Autodesk Inventor part; units mm, degrees
ref_plane "YZ Plane" through (0, 0, 0) normal (1, 0, 0) x (0, 1, 0)
ref_plane "XZ Plane" through (0, 0, 0) normal (0, 1, 0) x (-1, 0, 0)
ref_plane "XY Plane" through (0, 0, 0) normal (0, 0, 1) x (1, 0, 0)
sketch "Sketch1" plane through (0, 0, 0) normal (0, 1, 0) x (-1, 0, 0)
  circle A0 centre (0, 0) radius 2.54
  circle A1 centre (0, 0) radius 5.461
  dimension "d0" = 5.08
  dimension "d1" = 10.922
extrude "Extrusion1" add sketch "Sketch1" along normal blind 14.605 contours A0 | A1
sketch "Sketch2" plane through (0, 0, 0) normal (1, 0, 0) x (0, 1, 0)
  arc A0 (12.065, -2.54) -> (12.065, 2.54) centre (12.065, 0) ccw
  line L0 (0, 5.461) -> (14.605, 5.461)
  line L1 (0, -5.461) -> (14.605, -5.461)
  line L2 (12.065, 2.54) -> (7.1656, 2.54)
  line L3 (12.065, -2.54) -> (7.1656, -2.54)
  line L4 (4.6256, 5.461) -> (4.6256, 5.08)
  line L5 (4.6256, -5.08) -> (4.6256, -5.461)
  arc A1 (4.6256, 5.08) -> (7.1656, 2.54) centre (7.1656, 5.08) ccw
  arc A2 (7.1656, -2.54) -> (4.6256, -5.08) centre (7.1656, -5.08) ccw
  line L6 (14.605, 2.54) -> (14.605, -2.54)
  line L7 (14.605, -5.461) -> (14.605, 5.461)
  point P0 (0, 0)
  point P1 (14.605, 0)
  dimension "d4" = 2.54
  dimension "d5" = 2.54
extrude "Extrusion2" cut sketch "Sketch2" along normal mid plane 14.605
properties part number "Half Universal"
Verification items for the finished model (mm, model axes). A direction names the side the tool comes from. Round coordinates to 2 decimals unless told otherwise and drop trailing zeros. Write each loop counter-clockwise with the first axis right and the second up, starting at its lowest first coordinate (ties: lowest second). Pieces come first, ordered by that corner, then holes.
1. Section check B-B on y = 11.5. Enter the section's corners in (x, z).
2. Scan lines: L1, parallel to Z at x = 2, y = 3.5; L2, parallel to Z at x = 1.5, y = 11.5. Record each from-to range of solid material in increasing order.
3. Section check D-D on z = -3.5. Enter the section's corners in (x, y), plus the area to 3 significant figures.
4. Section check C-C on x = -2.5. Enter the section's corners in (y, z) (3 decimals), plus the area to 3 significant figures.
5. Section check A-A on x = 0. Enter the section's corners in (y, z) (3 decimals), plus the area to 3 significant figures.
6. Gauge pin test, flat ends, axial feed: P1, Ø6, axis at x = -1, z = 0.5, coming from the +Y side (3 decimals); P2, Ø6, axis at x = 4, y = 11, coming from the +Z side; P3, Ø1.5, axis at y = 12, z = -2, coming from the +X side; P4, Ø1, axis at y = 4, z = -2.5, coming from the +X side. Record the tip position at first contact, or that the pin passes through.
7. Access from +Z, -Z, +X, -X, +Y, -Y to the whole of each face (thin tool, end or side, straight path). Record for faces 1 (the flat face through (0, 0, 0)), 2 (the flat face through (0, 10, -2.54)), 3 (the flat face through (0, 10, 2.54)).
Answer:
1. outline: (-4.83, -2.54) - (4.83, -2.54) arc R5.46 ccw to (4.83, 2.54) - (-4.83, 2.54) arc R5.46 ccw to start
2. L1: z = -5.08 to 5.08
2. L2: z = -2.54 to 2.54
3. outline: (-4.19, 0) - (4.19, 0) - (4.19, 5.18) - (-4.19, 5.18) - close
3. area: 43.4 mm2
4. outline: (0, -4.855) - (4.636, -4.855) arc R2.54 cw to (7.166, -2.54) - (12.065, -2.54) arc R2.54 ccw to (12.065, 2.54) - (7.166, 2.54) arc R2.54 cw to (4.636, 4.855) - (0, 4.855) - close
4. area: 95.6 mm2
5. outline: (0, -5.461) - (4.626, -5.461) - (4.626, -5.08) arc R2.54 cw to (7.166, -2.54) - (12.065, -2.54) arc R2.54 ccw to (12.065, 2.54) - (7.166, 2.54) arc R2.54 cw to (4.626, 5.08) - (4.626, 5.461) - (0, 5.461) - close
5. area: 101 mm2
6. P1: stops at y = 14.605
6. P2: stops at z = 2.54
6. P3: stops at x = 5.32
6. P4: stops at x = 5.08
7. face 1: +Z, -Z, +X, -X, -Y
7. face 2: -Z, +X, -X, +Y
7. face 3: +Z, +X, -X, +Y
